```python
from build123d import *

# Parameters (mm, degrees)
SKETCH1_R           = 2.15
SKETCH1_R_2         = 3.5
SKETCH1_W           = 9.000072
SKETCH1_H           = 2
SKETCH1_W_2         = 5
BOSS_EXTRUDE1_DEPTH = 4
SKETCH2_W           = 8
SKETCH2_H           = 4
CUT_EXTRUDE1_DEPTH  = 5


with BuildPart() as part:
    # Sketch1 → Boss-Extrude1 (new body)
    with BuildSketch(Plane.XY):
        with BuildLine():
            Line((-12.978640908, -18), (-12.978640908, -24))
            Line((-12.978640908, -24), (23.021359092, -24))
            Line((23.021359092, -24), (23.021359092, -18))
            ThreePointArc((23.021359092, -18), (33.536808213, -15.187172163), (41.243562055, -7.5))
            ThreePointArc((41.243562055, -7.5), (47.269076761, 9.160930487), (49.313899811, 26.759570515))
            ThreePointArc((49.313899811, 26.759570515), (48.54170687, 46.985091914), (46.229623828, 67.092858318))
            Line((46.229623828, 67.092858318), (30.150376172, 69.067141682))
            Line((30.150376172, 69.067141682), (27.668766331, 75.523635508))
            Line((27.668766331, 75.523635508), (11.471233669, 75.806364492))
            Line((11.471233669, 75.806364492), (8.1, 82.51))
            Line((8.1, 82.51), (-8.1, 82.51))
            Line((-8.1, 82.51), (-15.746217975, 82.280462515))
            Line((-15.746217975, 82.280462515), (-31.943782025, 81.999537485))
            ThreePointArc((-31.943782025, 81.999537485), (-38.683922922, 47.231229605), (-38.032696315, 11.821617405))
            ThreePointArc((-38.032696315, 11.821617405), (-29.918009554, -6.796134249), (-12.978640908, -18))
        make_face()
        with Locations((38.147341743, 11.821617405)):
            Circle(SKETCH1_R, mode=Mode.SUBTRACT)
        with Locations((-24.678960076, 61.651218734)):
            Circle(SKETCH1_R_2, mode=Mode.SUBTRACT)
        with Locations((1.521420673, 61.651218734)):
            Circle(SKETCH1_R_2, mode=Mode.SUBTRACT)
        with Locations((14.86306514, 46.821617405)):
            Circle(SKETCH1_R_2, mode=Mode.SUBTRACT)
        with Locations((38.147341743, 46.821617405)):
            Circle(SKETCH1_R_2, mode=Mode.SUBTRACT)
        with Locations((-31.681501662, 43.456405989)):
            Circle(SKETCH1_R, mode=Mode.SUBTRACT)
        with Locations((0, 77.51)):
            Rectangle(SKETCH1_W, SKETCH1_H, mode=Mode.SUBTRACT)
        Polygon((-4, -2.5), (0, -2.5), (0, 0), (12, 0), (12, -2.5), (16, -2.5), (16, -12.5), (12, -12.5), (12, -15), (0, -15), (0, -12.5), (-4, -12.5), align=None, mode=Mode.SUBTRACT)
        with Locations((35.147341743, 56.321617405)):
            Rectangle(SKETCH1_W_2, SKETCH1_H, mode=Mode.SUBTRACT)
        Polygon((-28.274995137, 78.062566115), (-19.276276454, 78.218636824), (-19.241594351, 76.218937559), (-28.240313034, 76.062866849), align=None, mode=Mode.SUBTRACT)
        with Locations((17.86306514, 56.321617405)):
            Rectangle(SKETCH1_W_2, SKETCH1_H, mode=Mode.SUBTRACT)
        with Locations((-0.478579327, 71.151218734)):
            Rectangle(SKETCH1_W_2, SKETCH1_H, mode=Mode.SUBTRACT)
        Polygon((15.000839752, 71.744145677), (14.965934939, 69.744450286), (23.964636184, 69.587377372), (23.999540997, 71.587072762), align=None, mode=Mode.SUBTRACT)
        Polygon((42.16901604, 63.561398961), (33.236029212, 64.658231826), (32.992290526, 62.673139523), (41.925277354, 61.576306658), align=None, mode=Mode.SUBTRACT)
        Polygon((1.667459367, 35.705611754), (1.005748572, 29.742211816), (-18.872251222, 31.947914464), (-18.210540428, 37.911314402), align=None, mode=Mode.SUBTRACT)
        with Locations((-22.678960076, 71.151218734)):
            Rectangle(SKETCH1_W_2, SKETCH1_H, mode=Mode.SUBTRACT)
        Polygon((0.013182381, 20.797111909), (-1.310239208, 8.870312032), (-21.188239002, 11.076014679), (-19.864817414, 23.002814556), align=None, mode=Mode.SUBTRACT)
        Polygon((-10.203, 23.988271038), (-9.6615, 28.868319988), (-23.705306855, 30.426648908), (-23.264166325, 34.402248867), (-31.215366243, 35.284529926), (-31.656506773, 31.308929968), (-34.636711633, 31.639619464), (-35.178211633, 26.759570515), (-32.198006773, 26.428881018), (-32.639147302, 22.453281059), (-24.687947384, 21.571), (-24.246806855, 25.546599959), align=None, mode=Mode.SUBTRACT)
    extrude(amount=BOSS_EXTRUDE1_DEPTH)

    # Sketch2 → Cut-Extrude1 (cut, through all)
    with BuildSketch(Plane(origin=(0, 0, 0), x_dir=(-1, 0, 0), z_dir=(0, 0, -1))):
        with Locations((-28.271359092, -8)):
            Rectangle(SKETCH2_W, SKETCH2_H)
        with Locations((18.228640908, -8)):
            Rectangle(SKETCH2_W, SKETCH2_H)
    extrude(amount=-CUT_EXTRUDE1_DEPTH, mode=Mode.SUBTRACT)


solid = part.part
```
The listing builds one solid part. Answer for the finished solid, in the listing's coordinates (mm). A direction names the side the tool comes from. Give positions to 0.01 mm unless a question says otherwise; leave off trailing zeros. Write each loop counter-clockwise with the first axis right and the second up, starting at its lowest first coordinate (ties: lowest second). Pieces come first, ordered by that corner, then holes. Notation, with made-up numbers: (-23, -35) -> (14, -35) arc R15 ccw to (14, -24) -> close; hole circle Ø10 at (73, 87.25). An arc over 180 degrees is marked (long way). Write item = value, one per line. Start each with the question number.
1) The part is cut by section B-B, the plane z = 2.75. Count the separate pieces of the cut face and the enclosed holes in it, and give its area (3 significant figures).
2) The part is cut by section C-C, the plane y = 5. Determine the outline of the cut face in (x, z), and give its area (3 significant figures).
3) Determine the mould class of faces 1 (the face through (-12.979, -21, 2)), 2 (the face through (-10.065, 21.915, 1.972)), 3 (the face through (33.403, -15.264, 1.972)) for opening direction Y: +Y half, -Y half, draft (parallel to the pull), parting line (faces both ways), or undercut.
4) Straight lines are drawn through the part: line 1 along Y through (x, z) = (-17, 1.85); line 2 along Y through (x, z) = (19, 1.95); line 3 along Y through (x, z) = (17, 1.4). For each, find the intervals that lie inside material, in ascending order.
5) The part is cut by section A-A, the plane x = -27. Determine the outline of the cut face in (y, z).
6) Each of these flat-tipped pins is pushed along its axis until it touches: pin 1 (2 mm diameter, centred on y = 49.5, z = 3.5, fed in from +X); pin 2 (1.2 mm diameter, centred on x = 18, z = 2, fed in from +Y); pin 3 (1 mm diameter, centred on y = 71.5, z = 2, fed in from -X); pin 4 (4 mm diameter, centred on x = 14.86, y = 46.82, fed in from -Z). Where does it stop, or does it pass through?
7) Which of the six approach directions +Z, -Z, +X, -X, +Y, -Y give full straight-line access (tool end or side, diameter ignored) to faces 4 (the face through (23.021, -21, 2)), 5 (the face through (48.563, 46.702, 1.972)), 6 (the face through (-28.72, 22.02, 1.97))?
Solutions:
q1.separate_pieces = 1
q1.enclosed_holes = 20
q1.area = 6,860 mm²
q2.outline = (-36.5, 0) -> (46.16, 0) -> (46.16, 4) -> (-36.5, 4) -> close
q2.area = 331 mm²
q3.face_1 = draft
q3.face_2 = undercut
q3.face_3 = -Y half
q4.line_1 = -16.5 to -10, -6 to 10.61, 22.68 to 24.74, 29.68 to 31.74, 37.78 to 82.26
q4.line_2 = -24 to 55.32, 57.32 to 69.67, 71.67 to 75.67
q4.line_3 = -24 to 44.05, 49.59 to 55.32, 57.32 to 69.71, 71.71 to 75.71
q5.outline = (-9.88, 0) -> (21.83, 0) -> (21.83, 4) -> (-9.88, 4) -> close; (34.82, 0) -> (59.03, 0) -> (59.03, 4) -> (34.82, 4) -> close; (64.27, 0) -> (76.08, 0) -> (76.08, 4) -> (64.27, 4) -> close; (78.08, 0) -> (82.09, 0) -> (82.09, 4) -> (78.08, 4) -> close
q6.pin_1 = 48.42
q6.pin_2 = 75.7
q6.pin_3 = -34.9
q6.pin_4 = through
q7.face_4 = +Z, -Z, +X, -Y
q7.face_5 = +Z, -Z, +X, +Y
q7.face_6 = +Z, -Z
